Geometry: final body of the model. Coordinates: model frame, mm. A direction names the side the tool comes from. Round coordinates to 2 decimals unless told otherwise and drop trailing zeros. Loops run counter-clockwise (first coordinate to the right, second up) from the corner with the lowest first, then second, coordinate; pieces in that order, holes last. Notation, with made-up numbers: M -13.5,24.25 L 6.5,24.25 A26 ccw 6.5,44.25 Z; hole C -24.75,17 d1. An arc over 180 degrees is marked long. Answer as a JSON object with one key per item and string values.
from build123d import *

# Parameters (mm, degrees)
SKETCH1_W      = 43.18
SKETCH1_H      = 18.415
EXTRUDE1_DEPTH = 13.081
SKETCH2_R      = 0.769945783
SKETCH2_R_2    = 0.721607375
SKETCH2_R_3    = 0.762102327
SKETCH2_R_4    = 0.671282844
EXTRUDE2_DEPTH = 2.54
SKETCH4_W      = 9.3218
SKETCH4_H      = 8.001
EXTRUDE3_DEPTH = 4.0132


with BuildPart() as part:
    # Sketch1 → Extrude1 (new body)
    with BuildSketch(Plane.XY):
        Rectangle(SKETCH1_W, SKETCH1_H)
    extrude(amount=EXTRUDE1_DEPTH)

    # Sketch2 → Extrude2 (add)
    with BuildSketch(Plane(origin=(0, 0, 0), x_dir=(-1, 0, 0), z_dir=(0, 0, -1))):
        with Locations((-17.78, 7.62)):
            Circle(SKETCH2_R)
        with Locations((-17.78, -7.62)):
            Circle(SKETCH2_R_2)
        with Locations((17.78, -7.62)):
            Circle(SKETCH2_R_3)
        with Locations((17.78, 7.62)):
            Circle(SKETCH2_R_4)
    extrude(amount=EXTRUDE2_DEPTH)

    # Sketch4 → Extrude3 (add)
    with BuildSketch(Plane.XY.offset(13.081)):
        with Locations((-18.7579, 0)):
            Rectangle(SKETCH4_W, SKETCH4_H)
    extrude(amount=EXTRUDE3_DEPTH)


solid = part.part
1) Pull-direction query (Y, two-part tool) for faces 1 (the flat face through (-19, 0, 17.094)), 2 (the flat face through (0, 9.208, 6)), 3 (the cylindrical face through (-17.02, -7.59, -1.25)), 4 (the cylindrical face through (-18.42, 7.82, -1.25)); classes: +Y half, -Y half, draft (parallel to the pull), parting line (faces both ways), or undercut.
Results:
{"face 1": "draft", "face 2": "+Y half", "face 3": "undercut", "face 4": "undercut"}
2) Section query D-D (y = 2.5). Return the cut outline in (x, z).
Results:
{"outline": "M -23.42,13.08 L -21.59,13.08 L -21.59,0 L 21.59,0 L 21.59,13.08 L -14.1,13.08 L -14.1,17.09 L -23.42,17.09 Z"}
3) Section query C-C (z = 8.25). Return the cut outline in (x, y).
Results:
{"outline": "M -21.59,-9.21 L 21.59,-9.21 L 21.59,9.21 L -21.59,9.21 Z"}
4) Reachability of faces 5 (the flat face through (-19, 4, 15)), 6 (the cylindrical face through (18.55, 7.65, -1.25)), 7 (the flat face through (-14.097, 0, 15)), 8 (the flat face through (-23, 0, 13.081)) from +Z, -Z, +X, -X, +Y, -Y: full face, straight path, thin tool, end or side. Return the list, or none.
Results:
{"face 5": "+Z, +X, -X, +Y", "face 6": "-Z", "face 7": "+Z, +X, +Y, -Y", "face 8": "-Z, -X, +Y, -Y"}
5) Section query A-A (x = -17.78). Return the cut outline in (y, z), and give its area (3 significant figures).
Results:
{"outline": "M -9.21,0 L -8.38,0 L -8.38,-2.54 L -6.86,-2.54 L -6.86,0 L 6.95,0 L 6.95,-2.54 L 8.29,-2.54 L 8.29,0 L 9.21,0 L 9.21,13.08 L 4,13.08 L 4,17.09 L -4,17.09 L -4,13.08 L -9.21,13.08 Z", "area": "280 mm2"}
6) Ray query, line 1 (Z direction, x = 2.5, y = -5.75); line 2 (Z direction, x = -20.5, y = -3.75); line 3 (X direction, y = -6.75, z = 10.5). Return the intervals inside material, ascending.
Results:
{"line 1": "0 to 13.08", "line 2": "0 to 17.09", "line 3": "-21.59 to 21.59"}
7) Section query B-B (y = -7.62). Return the cut outline in (x, z).
Results:
{"outline": "M -21.59,0 L -18.54,0 L -18.54,-2.54 L -17.02,-2.54 L -17.02,0 L 17.06,0 L 17.06,-2.54 L 18.5,-2.54 L 18.5,0 L 21.59,0 L 21.59,13.08 L -21.59,13.08 Z"}
8) Pin query (flat end, axial travel): P1, Ø6, axis at x = -10, y = 6.5, coming from the +Z side; P2, Ø1, axis at x = -3.5, y = -0.5, coming from the -Z side; P3, Ø3, axis at x = -16.5, z = 16, coming from the -Y side; P4, Ø10, axis at y = -7, z = 9.5, coming from the -X side. Return the tip coordinate at first contact, or that it passes through.
Results:
{"P1": "z = 13.08", "P2": "z = 0", "P3": "y = -4", "P4": "x = -23.42"}
